Can you work these out from the model? Positions are in its coordinate system, mm. Face numbers are marked on the shaded views. A direction names the side the tool comes from. Round coordinates to 2 decimals unless told otherwise and drop trailing zeros. Loops run counter-clockwise (first coordinate to the right, second up) from the corner with the lowest first, then second, coordinate; pieces in that order, holes last. Notation, with made-up numbers: (50, 78.5) - (62, 78.5) arc R29 cw to (62, 108.5) - close; hole circle Ø3 at (18.5, 51). An arc over 180 degrees is marked (long way). Answer as CSV lines item,"result".
```python
from build123d import *

# Parameters (mm, degrees)
F0_R     = 1.25
F1_DEPTH = 3


with BuildPart() as f1:
    # F0 (on Right) → F1 (new body)
    with BuildSketch(Plane.YZ):
        with BuildLine():
            Line((-11.9511362031, -5.3111244172), (-11.9511362031, -13.7053132072))
            Line((-11.9511362031, -13.7053132072), (6.35, -13.7053132072))
            Line((6.35, -13.7053132072), (6.35, -6.9134512067))
            Line((6.35, -6.9134512067), (-0.8936743198, -6.9134512067))
            Line((-0.8936743198, -6.9134512067), (-2.7451495133, -7.2361294001))
            ThreePointArc((-2.7451495133, -7.2361294001), (-3.9259868399, -7.5186674947), (-5.1327843279, -7.6522503891))
            ThreePointArc((-5.1327843279, -7.6522503891), (-8.7662829798, -7.1350102989), (-11.9511362031, -5.3111244172))
        make_face()
        with Locations((-6.35, -10.0884512067)):
            Circle(F0_R, mode=Mode.SUBTRACT)
        with Locations((0, -10.0884512067)):
            Circle(F0_R, mode=Mode.SUBTRACT)
        with BuildLine():
            ThreePointArc((-5.1327843279, 11.8253479758), (-14.6592384736, 5.6910873598), (-11.9511362031, -5.3111244172))
            ThreePointArc((-11.9511362031, -5.3111244172), (-8.7662829798, -7.1350102989), (-5.1327843279, -7.6522503891))
            Line((-5.1327843279, -7.6522503891), (-2.7451495133, -7.2361294001))
            ThreePointArc((-2.7451495133, -7.2361294001), (-1.3343098737, -6.6807990238), (-0.0266257976, -5.9134512067))
            Line((-0.0266257976, -5.9134512067), (-2.9884921599, -6.2646503302))
            ThreePointArc((-2.9884921599, -6.2646503302), (-7.3981085591, -6.4767044208), (-11.35, -4.5089041858))
            ThreePointArc((-11.35, -4.5089041858), (-14.35, 2.0865487933), (-11.35, 8.6820017725))
            ThreePointArc((-11.35, 8.6820017725), (-7.3981085591, 10.6498020075), (-2.9884921599, 10.4377479169))
            Line((-2.9884921599, 10.4377479169), (-0.0266257976, 10.0865487933))
            ThreePointArc((-0.0266257976, 10.0865487933), (-1.3343098737, 10.8538966105), (-2.7451495133, 11.4092269868))
            Line((-2.7451495133, 11.4092269868), (-5.1327843279, 11.8253479758))
        make_face()
        with BuildLine():
            ThreePointArc((-2.7451495133, 11.4092269868), (-3.9259868399, 11.6917650813), (-5.1327843279, 11.8253479758))
            Line((-5.1327843279, 11.8253479758), (-2.7451495133, 11.4092269868))
        make_face()
        with BuildLine():
            Line((-0.8936743198, -6.9134512067), (6.35, -6.9134512067))
            Line((6.35, -6.9134512067), (6.35, -3.945808849))
            Line((6.35, -3.945808849), (5.35, -3.945808849))
            Line((5.35, -3.945808849), (5.35, -5.9134512067))
            Line((5.35, -5.9134512067), (-0.0266257976, -5.9134512067))
            ThreePointArc((-0.0266257976, -5.9134512067), (-1.3343098737, -6.6807990238), (-2.7451495133, -7.2361294001))
            Line((-2.7451495133, -7.2361294001), (-0.8936743198, -6.9134512067))
        make_face()
        with BuildLine():
            Line((-0.8936743198, 11.0865487933), (-2.7451495133, 11.4092269868))
            ThreePointArc((-2.7451495133, 11.4092269868), (-1.3343098737, 10.8538966105), (-0.0266257976, 10.0865487933))
            Line((-0.0266257976, 10.0865487933), (5.35, 10.0865487933))
            Line((5.35, 10.0865487933), (5.35, 8.1189064356))
            Line((5.35, 8.1189064356), (6.35, 8.1189064356))
            Line((6.35, 8.1189064356), (6.35, 11.0865487933))
            Line((6.35, 11.0865487933), (-0.8936743198, 11.0865487933))
        make_face()
        Polygon((5.35, -3.945808849), (6.35, -3.945808849), (6.35, 2.0865487933), (6.35, 8.1189064356), (5.35, 8.1189064356), (5.35, 2.0865487933), align=None)
        with BuildLine():
            ThreePointArc((4.15, 2.0865487933), (3.0430000137, 6.5988708965), (-0.0266257976, 10.0865487933))
            Line((-0.0266257976, 10.0865487933), (-2.9884921599, 10.4377479169))
            ThreePointArc((-2.9884921599, 10.4377479169), (-1.328072511, 9.7228525804), (0.15, 8.6820017725))
            ThreePointArc((0.15, 8.6820017725), (2.364766161, 5.7093929799), (3.15, 2.0865487933))
            ThreePointArc((3.15, 2.0865487933), (2.364766161, -1.5362953932), (0.15, -4.5089041858))
            ThreePointArc((0.15, -4.5089041858), (-1.328072511, -5.5497549938), (-2.9884921599, -6.2646503302))
            Line((-2.9884921599, -6.2646503302), (-0.0266257976, -5.9134512067))
            ThreePointArc((-0.0266257976, -5.9134512067), (3.0430000137, -2.4257733099), (4.15, 2.0865487933))
        make_face()
        with BuildLine():
            Line((5.35, 10.0865487933), (-0.0266257976, 10.0865487933))
            ThreePointArc((-0.0266257976, 10.0865487933), (3.0430000137, 6.5988708965), (4.15, 2.0865487933))
            ThreePointArc((4.15, 2.0865487933), (3.0430000137, -2.4257733099), (-0.0266257976, -5.9134512067))
            Line((-0.0266257976, -5.9134512067), (5.35, -5.9134512067))
            Line((5.35, -5.9134512067), (5.35, -3.945808849))
            Line((5.35, -3.945808849), (5.35, 2.0865487933))
            Line((5.35, 2.0865487933), (5.35, 8.1189064356))
            Line((5.35, 8.1189064356), (5.35, 10.0865487933))
        make_face()
        with BuildLine():
            Line((-11.35, -4.5089041858), (-11.35, 8.6820017725))
            ThreePointArc((-11.35, 8.6820017725), (-14.35, 2.0865487933), (-11.35, -4.5089041858))
        make_face()
        with BuildLine():
            ThreePointArc((3.15, 2.0865487933), (2.364766161, 5.7093929799), (0.15, 8.6820017725))
            Line((0.15, 8.6820017725), (0.15, -4.5089041858))
            ThreePointArc((0.15, -4.5089041858), (2.364766161, -1.5362953932), (3.15, 2.0865487933))
        make_face()
        with BuildLine():
            Line((-2.7451495133, -7.2361294001), (-5.1327843279, -7.6522503891))
            ThreePointArc((-5.1327843279, -7.6522503891), (-3.9259868399, -7.5186674947), (-2.7451495133, -7.2361294001))
        make_face()
    extrude(amount=F1_DEPTH)


solid = f1.part
```
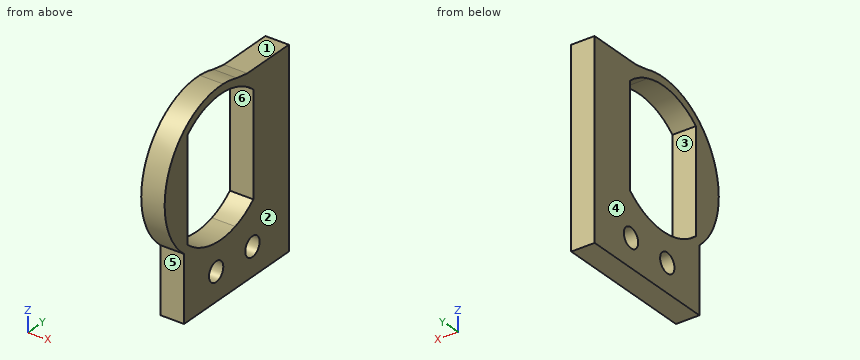
Q1. Imagine slicing it at D-D (x = 0.75). Write out the boundary of the cut face in (y, z), then the cut area to 3 significant figures.
Checks:
outline,"(-11.95, -13.71) - (6.35, -13.71) - (6.35, 11.09) - (-0.89, 11.09) - (-2.75, 11.41) arc R9.75 ccw to (-11.95, -5.31) - close; hole (-11.35, -4.51) arc R8.75 ccw to (0.15, -4.51) - (0.15, 8.68) arc R8.75 ccw to (-11.35, 8.68) - close; hole circle Ø2.5 at (-6.35, -10.09); hole circle Ø2.5 at (0, -10.09)"
area,"295 mm²"
Q2. Imagine slicing it at C-C (y = -4). Write out the boundary of the cut face in (x, z), then the cut area to 3 significant figures.
Checks:
outline,"(0, -13.71) - (3, -13.71) - (3, -6.52) - (0, -6.52) - close; (0, 10.69) - (3, 10.69) - (3, 11.7) - (0, 11.7) - close"
area,"24.6 mm²"
Q3. I'm going to push flat-ended pins straight in: pin 1 Ø1 at (x, y) = (1.5, 3.5) entering from +Z; pin 2 Ø1.5 at (x, z) = (1, 4.5) entering from -Y. Where does each tip first touch, or does it pass through?
Checks:
pin 1,"z = 11.09"
pin 2,"y = -15.21"
Q4. If I drill on line 1 along Z through (x, y) = (0.75, -6.35); line 2 along Z through (x, y) = (2.05, -0.25); line 3 along Z through (x, y) = (0.5, 3.75), over which ranges is the centre line in solid material (lowest first)? Write a range as [from, to].
Checks:
line 1,"[-13.71, -11.34], [-8.84, -6.63], [10.8, 11.81]"
line 2,"[-13.71, -11.31], [-8.86, -4.84], [9.01, 11.09]"
line 3,"[-13.71, 11.09]"
Q5. Imagine slicing it at A-A (z = -2.5). Write out the boundary of the cut face in (x, y), then the cut area to 3 significant figures.
Checks:
outline,"(0, -14.2) - (3, -14.2) - (3, -11.35) - (0, -11.35) - close; (0, 0.15) - (3, 0.15) - (3, 6.35) - (0, 6.35) - close"
area,"27.2 mm²"
Q6. We'd pull the mould along Z, two halves only. Please class the marked faces 1, 2 and 3: pulls with the +Z half, pulls with the -Z half, needs draft (parallel to the pull), parting line crosses it, or undercut.
Checks:
face 1,"pulls with the +Z half"
face 2,"needs draft"
face 3,"undercut"
Q7. Imagine slicing it at B-B (y = -6.35). Write out the boundary of the cut face in (x, z), then the cut area to 3 significant figures.
Checks:
outline,"(0, -13.71) - (3, -13.71) - (3, -11.34) - (0, -11.34) - close; (0, -8.84) - (3, -8.84) - (3, -6.63) - (0, -6.63) - close; (0, 10.8) - (3, 10.8) - (3, 11.81) - (0, 11.81) - close"
area,"16.7 mm²"
Q8. On a 3-axis mill with a long thin cutter (end or side, diameter ignored), from which of +Z, -Z, +X, -X, +Y, -Y can I reach the whole of each face in a straight line? I mean the marked faces 4, 5 and 6. Say none if no direction works.
Checks:
face 4,"+Z, -Z, -X, +Y, -Y"
face 5,"-Z, +X, -X, -Y"
face 6,"+X, -X"
